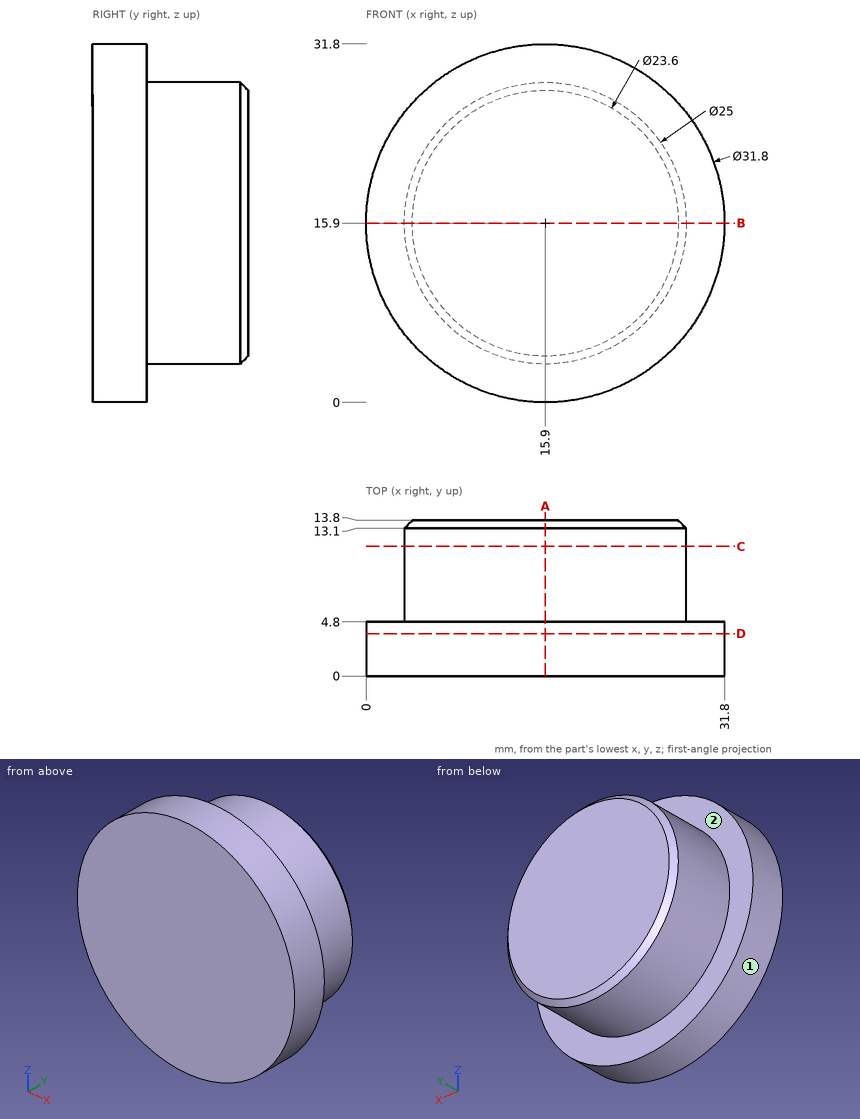
Geometry check sheet. Reference: drawing and pictorial views, mm from the part's lowest x, y, z. A direction names the side the tool comes from. Give positions to 0.01 mm unless a question says otherwise; leave off trailing zeros. Write each loop counter-clockwise with the first axis right and the second up, starting at its lowest first coordinate (ties: lowest second). Pieces come first, ordered by that corner, then holes.
Item 1: Access from +Z, -Z, +X, -X, +Y, -Y to the whole of each face (thin tool, end or side, straight path). Record for the marked faces 1 and 2.
Item 2: Scan lines: L1, parallel to Y at x = 22, z = 4; L2, parallel to X at y = 13, z = 10; L3, parallel to X at y = 8.5, z = 7.5. Record each from-to range of solid material in increasing order.
Item 3: Cross-section at C-C (y = 11.5). Enter the section's corners in (x, z), and give its area (3 significant figures).
Item 4: Cross-section at D-D (y = 3.75). Enter the section's corners in (x, z), and give its area (3 significant figures).
Item 5: Cross-section at B-B (z = 15.9). Enter the section's corners in (x, y), and give its area (3 significant figures).
Item 6: Gauge pin test, flat ends, axial feed: pin 1 (6 mm diameter, centred on x = 21.5, y = 11.5, fed in from -Z); pin 2 (1.5 mm diameter, centred on y = 4, z = 19.5, fed in from -X); pin 3 (8 mm diameter, centred on x = 6, y = 11.5, fed in from +Z). Record the tip position at first contact, or that the pin passes through.
Item 7: Cross-section at A-A (x = 15.9). Enter the section's corners in (y, z).
Report:
1. face 1: +Y, -Y
1. face 2: +Y
2. L1: y = 0 to 4.8
2. L2: x = 4.88 to 26.92
2. L3: x = 6.64 to 25.16
3. outline: circle Ø25 at (15.9, 15.9)
3. area: 491 mm2
4. outline: circle Ø31.8 at (15.9, 15.9)
4. area: 794 mm2
5. outline: (0, 0) - (31.8, 0) - (31.8, 4.8) - (28.4, 4.8) - (28.4, 13.1) - (27.7, 13.8) - (4.1, 13.8) - (3.4, 13.1) - (3.4, 4.8) - (0, 4.8) - close
5. area: 377 mm2
6. pin 1: stops at z = 3.67
6. pin 2: stops at x = 0.26
6. pin 3: stops at z = 26.92
7. outline: (0, 0) - (4.8, 0) - (4.8, 3.4) - (13.1, 3.4) - (13.8, 4.1) - (13.8, 27.7) - (13.1, 28.4) - (4.8, 28.4) - (4.8, 31.8) - (0, 31.8) - close
